```python
from build123d import *

# Parameters (mm, degrees)
ESQUISSE1_W             = 10.2
ESQUISSE1_H             = 15.1
ESQUISSE1_R             = 1.85
BOSS_EXTRU_1_DEPTH      = 1.27
ESQUISSE2_W             = 10.2
ESQUISSE2_H             = 8.6
BOSS_EXTRU_2_DEPTH      = 3.18
ENL_V_MAT_EXTRU_1_DEPTH = 11.944062317
ENL_V_MAT_EXTRU_2_DEPTH = 19.757731739
ESQUISSE5_W             = 1.5
ESQUISSE5_H             = 0.5
BOSS_EXTRU_3_DEPTH      = 3.1
ESQUISSE6_W             = 0.8
ESQUISSE6_H             = 0.5
BOSS_EXTRU_4_DEPTH      = 3.5
CHANFREIN1_SIZE         = 0.35
CHANFREIN2_SIZE         = 1
ESQUISSE8_W             = 1.27
ESQUISSE8_H             = 5.5
ENL_V_MAT_EXTRU_4_DEPTH = 0.01
ESQUISSE9_W             = 1.27
ESQUISSE9_H             = 5.5
ENL_V_MAT_EXTRU_5_DEPTH = 0.01
BOSS_EXTRU_6_DEPTH      = 0.01


with BuildPart() as part:
    # Esquisse1 → Boss.-Extru.1 (new body)
    with BuildSketch(Plane.XY):
        with Locations((0, 7.55)):
            Rectangle(ESQUISSE1_W, ESQUISSE1_H)
        with Locations((0, 12.36)):
            Circle(ESQUISSE1_R, mode=Mode.SUBTRACT)
    extrude(amount=BOSS_EXTRU_1_DEPTH)

    # Esquisse2 → Boss.-Extru.2 (add)
    with BuildSketch(Plane.XY.offset(1.27)):
        with Locations((0, 4.3)):
            Rectangle(ESQUISSE2_W, ESQUISSE2_H)
    extrude(amount=BOSS_EXTRU_2_DEPTH)

    # Esquisse3 → Enlèv. mat.-Extru.1 (cut, through all)
    with BuildSketch(Plane(origin=(0, 8.6, 0), x_dir=(1, 0, 0), z_dir=(0, 1, 0))):
        Polygon((5.1, -1.27), (4.9, -4.45), (5.1, -4.45), align=None)
        Polygon((-5.1, -1.27), (-5.1, -4.45), (-4.9, -4.45), align=None)
    extrude(amount=-ENL_V_MAT_EXTRU_1_DEPTH, mode=Mode.SUBTRACT)

    # Esquisse4 → Enlèv. mat.-Extru.2 (cut, through all)
    with BuildSketch(Plane(origin=(5.1, 0, 0), x_dir=(0, 0, -1), z_dir=(1, 0, 0))):
        Polygon((-1.27, 8.6), (-4.45, 8.1), (-4.45, 8.6), align=None)
    extrude(amount=-ENL_V_MAT_EXTRU_2_DEPTH, mode=Mode.SUBTRACT)

    # Esquisse5 → Boss.-Extru.3 (add)
    with BuildSketch(Plane.XZ):
        with Locations((0, 3)):
            Rectangle(ESQUISSE5_W, ESQUISSE5_H)
        with Locations((2.54, 3)):
            Rectangle(ESQUISSE5_W, ESQUISSE5_H)
        with Locations((-2.54, 3)):
            Rectangle(ESQUISSE5_W, ESQUISSE5_H)
    extrude(amount=BOSS_EXTRU_3_DEPTH)

    # Esquisse6 → Boss.-Extru.4 (add)
    with BuildSketch(Plane.XZ.offset(3.1)):
        with Locations((-2.54, 3)):
            Rectangle(ESQUISSE6_W, ESQUISSE6_H)
        with Locations((0, 3)):
            Rectangle(ESQUISSE6_W, ESQUISSE6_H)
        with Locations((2.54, 3)):
            Rectangle(ESQUISSE6_W, ESQUISSE6_H)
    extrude(amount=BOSS_EXTRU_4_DEPTH)

    # Chanfrein1
    chanfrein1_edges = [part.edges().sort_by_distance(p)[0] for p in [
        (2.94, -3.1, 3),
        (0.4, -3.1, 3),
        (-2.14, -3.1, 3),
        (2.14, -3.1, 3),
        (-0.4, -3.1, 3),
        (-2.94, -3.1, 3),
    ]]
    chamfer(chanfrein1_edges, length=CHANFREIN1_SIZE - 0.0001)  # a hair under: the kernel refuses the full size

    # Chanfrein2
    chanfrein2_edges = [part.edges().sort_by_distance(p)[0] for p in [
        (-5.1, 15.1, 0.635),
        (5.1, 15.1, 0.635),
    ]]
    chamfer(chanfrein2_edges, length=CHANFREIN2_SIZE)

    # Esquisse8 → Enlèv. mat.-Extru.4 (cut)
    with BuildSketch(Plane(origin=(5.1, 0, 0), x_dir=(0, 0, -1), z_dir=(1, 0, 0))):
        with Locations((-0.635, 11.35)):
            Rectangle(ESQUISSE8_W, ESQUISSE8_H)
    extrude(amount=-ENL_V_MAT_EXTRU_4_DEPTH, mode=Mode.SUBTRACT)

    # Esquisse9 → Enlèv. mat.-Extru.5 (cut)
    with BuildSketch(Plane.ZY.offset(5.1)):
        with Locations((0.635, 11.35)):
            Rectangle(ESQUISSE9_W, ESQUISSE9_H)
    extrude(amount=-ENL_V_MAT_EXTRU_5_DEPTH, mode=Mode.SUBTRACT)

    # Esquisse11 → Boss.-Extru.6 (add)
    with BuildSketch(Plane(origin=(0, 0, 0), x_dir=(-1, 0, 0), z_dir=(0, 0, -1))):
        Polygon((-5.1, 0), (-5.1, 8.6), (-3.6, 8.6), (-3.6, 2), (3.59, 2), (3.59, 8.6), (5.09, 8.6), (5.1, 0), align=None)
    extrude(amount=BOSS_EXTRU_6_DEPTH)


solid = part.part
```
Could you check a few things on this model? Use its own coordinates, in mm. A direction names the side the tool comes from. Give positions to 0.01 mm unless a question says otherwise; leave off trailing zeros. Order: outer loops, then holes, each group sorted by start corner. A loop starts at its lowest first (then second) coordinate and runs counter-clockwise, first axis right, second up.
Q1. I'm going to push flat-ended pins straight in: P1, Ø1.4, axis at y = 11, z = 1, coming from the -X side; P2, Ø1.6, axis at x = 2.5, y = -2.5, coming from the +Z side; P3, Ø0.8, axis at x = -0.5, y = -3, coming from the -Z side. Where does each tip first touch, or does it pass through?
Q2. We'd pull the mould along X, two halves only. Please class faces 4 (the cylindrical face through (-0.401, 10.554, 0.626)), 5 (the flat face through (5.1, 4, 1)): +X half, -X half, draft (parallel to the pull), parting line (faces both ways), or undercut.
Q3. Suppose I cut it at D-D, the plane y = 12.36. Write out the boundary of the cut face in (x, z).
Q4. For faces 1 (the flat face through (-5, 4.36, 2.88)), 2 (the flat face through (-3, -3, 2.75)), 3 (the flat face through (-3, -3, 3.25)), which set-ups out of +Z, -Z, +X, -X, +Y, -Y let a thin tool reach every point of the face, with its end or its side?
Q5. If I drill on line 1 along Y through (x, z) = (0, 0.8); line 2 along Z through (x, y) = (-0.75, 6.25); line 3 along Z through (x, y) = (2.5, -4.5), over which ranges is the centre line in solid material (lowest first)?
Q6. Suppose I cut it at B-B, the plane y = -3.75. Write out the boundary of the cut face in (x, z), and give its area (3 significant figures).
Solution:
1. P1: stops at x = -5.09
1. P2: stops at z = 3.25
1. P3: stops at z = 2.75
2. face 4: undercut
2. face 5: +X half
3. outline: (-5.09, 0) - (-1.85, 0) - (-1.85, 1.27) - (-5.09, 1.27) - close; (1.85, 0) - (5.09, 0) - (5.09, 1.27) - (1.85, 1.27) - close
4. face 1: +Z, -X, +Y, -Y
4. face 2: -Z, +X, -X, -Y
4. face 3: +Z, +X, -X, -Y
5. line 1: y = 0 to 10.51, 14.21 to 15.1
5. line 2: z = 0 to 4.45
5. line 3: z = 2.75 to 3.25
6. outline: (-2.94, 2.75) - (-2.14, 2.75) - (-2.14, 3.25) - (-2.94, 3.25) - close; (-0.4, 2.75) - (0.4, 2.75) - (0.4, 3.25) - (-0.4, 3.25) - close; (2.14, 2.75) - (2.94, 2.75) - (2.94, 3.25) - (2.14, 3.25) - close
6. area: 1.20 mm2
